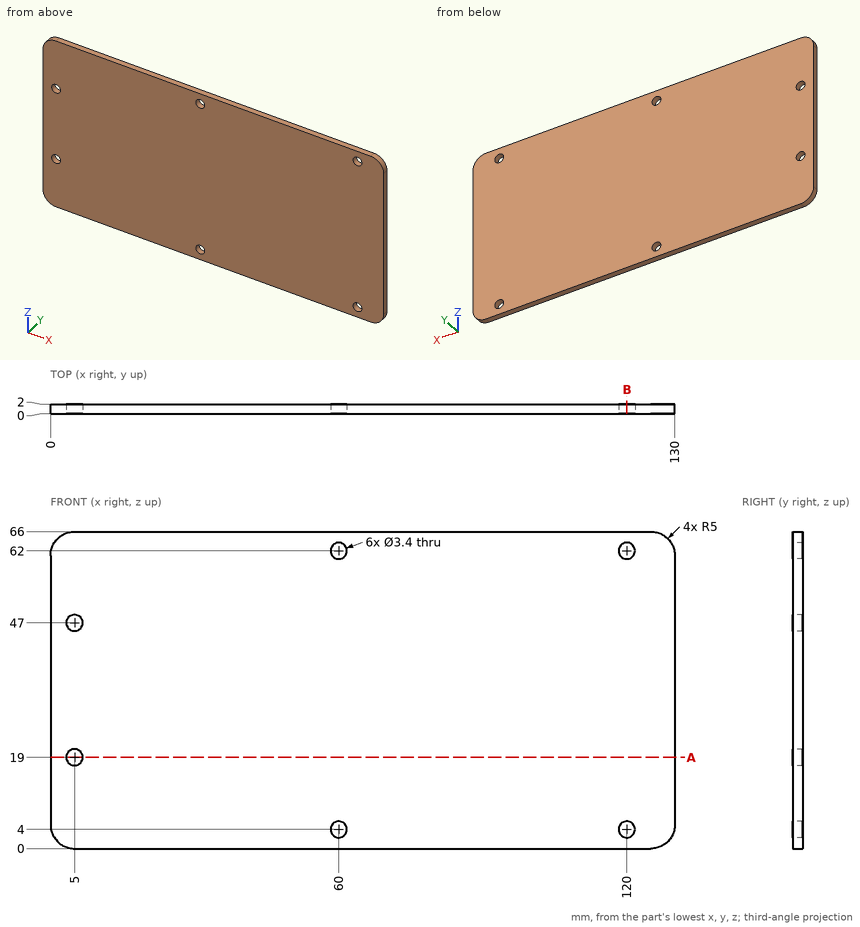
Input: dimensioned drawing with shaded views. Units: mm. Origin: part minimum x, y, z. Coordinates: 2 decimals unless noted, no trailing zeros. Order: outer loops, then holes, each group sorted by start corner. A loop starts at its lowest first (then second) coordinate and runs counter-clockwise, first axis right, second up. Notation, with made-up numbers: M -9,-1.75 L 49,-1.75 A20 cw 49,29.25 Z; hole C -5,65.25 d4. An arc over 180 degrees is marked long. Answer as CSV lines item,"result".
Q1. Line query: probe 1 along Z at (x, y) = (5, 0.65); probe 2 along Z at (x, y) = (120, 0.4); probe 3 along X at (y, z) = (1.9, 4). Output: solid intervals per line, ascending. Write a range as [from, to].
Answers:
probe 1,"z = [0, 17.3], [20.7, 45.3], [48.7, 66]"
probe 2,"z = [0, 2.3], [5.7, 60.3], [63.7, 66]"
probe 3,"x = [0.1, 58.3], [61.7, 118.3], [121.7, 129.9]"
Q2. Section A-A on z = 19. Return the cut outline in (x, y), and give its area (3 significant figures).
Answers:
outline,"M 0,0 L 3.3,0 L 3.3,2 L 0,2 Z; M 6.7,0 L 130,0 L 130,2 L 6.7,2 Z"
area,"253 mm^2"
Q3. Section B-B on x = 120. Return the cut outline in (y, z).
Answers:
outline,"M 0,0 L 2,0 L 2,2.3 L 0,2.3 Z; M 0,5.7 L 2,5.7 L 2,60.3 L 0,60.3 Z; M 0,63.7 L 2,63.7 L 2,66 L 0,66 Z"
Q4. First-contact query: P1, Ø2.5, axis at x = 5, z = 19, coming from the +Y side. Flat tip, straight axial feed; report the tip coordinate or a pass-through.
Answers:
P1,"passes through"
